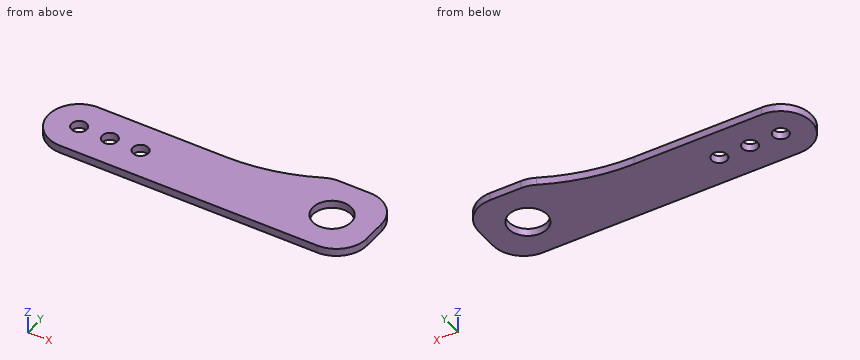
```python
from build123d import *

# Parameters (mm, degrees)
BOSS_EXTRUDE1_DEPTH = 2
SKETCH2_R           = 2
CUT_EXTRUDE1_DEPTH  = 2
SKETCH3_R           = 5
CUT_EXTRUDE2_DEPTH  = 2


with BuildPart() as part:
    # Sketch1 → Boss-Extrude1 (new body)
    with BuildSketch(Plane.XY):
        with BuildLine():
            Line((0, 8), (33.251315826, 8))
            ThreePointArc((33.251315826, 8), (44.62278648, 9.310271564), (55.398268548, 13.172413793))
            ThreePointArc((55.398268548, 13.172413793), (57.122345679, 13.79035655), (58.941780983, 14))
            Line((58.941780983, 14), (67, 14))
            ThreePointArc((67, 14), (72.656854249, 11.656854249), (75, 6))
            Line((75, 6), (75, 0))
            ThreePointArc((75, 0), (72.656854249, -5.656854249), (67, -8))
            Line((67, -8), (0, -8))
            ThreePointArc((0, -8), (-8, 0), (0, 8))
        make_face()
    extrude(amount=BOSS_EXTRUDE1_DEPTH)

    # Sketch2 → Cut-Extrude1 (cut)
    with BuildSketch(Plane.XY.offset(2)):
        Circle(SKETCH2_R)
        with Locations((8, 0)):
            Circle(SKETCH2_R)
        with Locations((16, 0)):
            Circle(SKETCH2_R)
    extrude(amount=-CUT_EXTRUDE1_DEPTH, mode=Mode.SUBTRACT)

    # Sketch3 → Cut-Extrude2 (cut)
    with BuildSketch(Plane.XY.offset(2)):
        with Locations((64, 3)):
            Circle(SKETCH3_R)
    extrude(amount=-CUT_EXTRUDE2_DEPTH, mode=Mode.SUBTRACT)


solid = part.part
```
Can you work these out from the model? Positions are in its coordinate system, mm. Round coordinates to 2 decimals unless told otherwise and drop trailing zeros. Loops run counter-clockwise (first coordinate to the right, second up) from the corner with the lowest first, then second, coordinate; pieces in that order, holes last.
Item 1: Suppose I cut it at A-A, the plane x = 64. Write out the boundary of the cut face in (y, z), then the cut area to 3 significant figures.
Item 2: Suppose I cut it at B-B, the plane z = 1.2. Write out the boundary of the cut face in (x, y).
Item 3: Will these pins go through, and if not, where does the flat tip stop? pin 1 Ø6.5 at (x, y) = (0, 0) entering from +Z; pin 2 Ø0.6 at (x, z) = (13, 0.5) entering from +Y.
Item 4: Suppose I cut it at C-C, the plane y = 3. Write out the boundary of the cut face in (x, z).
Item 5: Suppose I cut it at D-D, the plane x = 25.5. Write out the boundary of the cut face in (y, z), then the cut area to 3 significant figures.
Item 6: Please list where these lines run through material, in increasing order: L1, parallel to Y at x = 0, z = 0.7; L2, parallel to Y at x = 64, z = 1.15; L3, parallel to X at y = 0.25, z = 1.9.
Reported:
1. outline: (-8, 0) - (-2, 0) - (-2, 2) - (-8, 2) - close; (8, 0) - (14, 0) - (14, 2) - (8, 2) - close
1. area: 24.0 mm2
2. outline: (0, -8) - (67, -8) arc R8 ccw to (75, 0) - (75, 6) arc R8 ccw to (67, 14) - (58.94, 14) arc R8 ccw to (55.4, 13.17) arc R50 cw to (33.25, 8) - (0, 8) arc R8 ccw to start; hole circle Ø4 at (0, 0); hole circle Ø4 at (8, 0); hole circle Ø4 at (16, 0); hole circle Ø10 at (64, 3)
3. pin 1: stops at z = 2
3. pin 2: stops at y = 8
4. outline: (-7.42, 0) - (59, 0) - (59, 2) - (-7.42, 2) - close; (69, 0) - (75, 0) - (75, 2) - (69, 2) - close
5. outline: (-8, 0) - (8, 0) - (8, 2) - (-8, 2) - close
5. area: 32.0 mm2
6. L1: y = -8 to -2, 2 to 8
6. L2: y = -8 to -2, 8 to 14
6. L3: x = -8 to -1.98, 1.98 to 6.02, 9.98 to 14.02, 17.98 to 59.82, 68.18 to 75
